```python
from build123d import *

# Parameters (mm, degrees)
SKETCH2_R      = 12.7
EXTRUDE1_DEPTH = 12.7


with BuildPart() as part:
    # Sketch2 → Extrude1 (new, symmetric)
    with BuildSketch(Plane.XY):
        Polygon((0, -28.575), (0, -66.675), (76.2, -85.725), (76.2, -123.825), (-114.3, -123.825), (-114.3, -85.725), (-38.1, 28.575), (28.575, 28.575), (28.575, -28.575), align=None)
        with Locations(Location((0, 0, 0), (0, 0, 180))):
            Circle(SKETCH2_R, mode=Mode.SUBTRACT)
    extrude(amount=EXTRUDE1_DEPTH, both=True)


solid = part.part
```
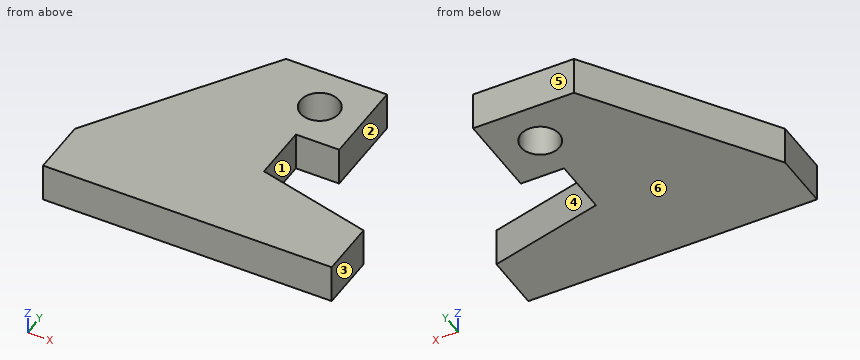
Design review of the part built by this model. Coordinates are the model's own, in mm. Face numbers are marked on the shaded views. A direction names the side the tool comes from. Give positions to 0.01 mm unless a question says otherwise; leave off trailing zeros. Order: outer loops, then holes, each group sorted by start corner. A loop starts at its lowest first (then second) coordinate and runs counter-clockwise, first axis right, second up. Notation, with made-up numbers: (-30, 63) -> (28, 63) arc R13 cw to (28, 67) -> close; hole circle Ø3 at (-36, 22). An arc over 180 degrees is marked (long way). Write item = value, one per line. Start each with the question number.
(1) We need section C-C on x = -4.5. Write out the cut boundary in (y, z) (3 decimals), plus the area to 3 significant figures.
(2) We need section D-D on y = -75. Write out the cut boundary in (x, z).
(3) To check wall thickness, follow line 1 along X through (y, z) = (2, 2.25) (3 decimals); line 2 along X through (y, z) = (7, -2.25) (3 decimals); line 3 along Y through (x, z) = (-94, 0) (3 decimals). State the ranges of each line that lie inside material, in increasing order.
(4) We need section A-A on z = 9.75. Write out the cut boundary in (x, y) (3 decimals).
(5) Mouldability with a two-part tool opening along Y and no side actions: class the marked faces 4, 5 and 6 as +Y half, -Y half, draft (parallel to the pull), parting line (faces both ways), or undercut.
(6) For the marked faces 1, 2 and 3, list the 3-axis set-ups (+Z, -Z, +X, -X, +Y, -Y) from which the entire face can be reached by the end or side of a thin tool; tool diameter is ignored.
(7) We need section B-B on y = 0. Write out the cut boundary in (x, z) (3 decimals), plus the area to 3 significant figures.
(8) For pin 1 (12 mm diameter, centred on x = -75.5, z = -3, fed in from +Y) (3 decimals); pin 2 (2 mm diameter, centred on y = -55, z = 3, fed in from -X); pin 3 (1.5 mm diameter, centred on x = -54, z = 10, fed in from +Y), all flat-tipped, find the tip position at first contact; note any pin that passes through.
Numbers:
q1.outline = (-123.825, -12.7) -> (-11.876, -12.7) -> (-11.876, 12.7) -> (-123.825, 12.7) -> close; (11.876, -12.7) -> (28.575, -12.7) -> (28.575, 12.7) -> (11.876, 12.7) -> close
q1.area = 3,270 mm^2
q2.outline = (-107.15, -12.7) -> (33.3, -12.7) -> (33.3, 12.7) -> (-107.15, 12.7) -> close
q3.line_1 = -55.817 to -12.542, 12.542 to 28.575
q3.line_2 = -52.483 to -10.597, 10.597 to 28.575
q3.line_3 = -123.825 to -55.275
q4.outline = (-114.3, -123.825) -> (76.2, -123.825) -> (76.2, -85.725) -> (0, -66.675) -> (0, -28.575) -> (28.575, -28.575) -> (28.575, 28.575) -> (-38.1, 28.575) -> (-114.3, -85.725) -> close; hole circle Ø25.4 at (0, 0)
q5.face_4 = undercut
q5.face_5 = +Y half
q5.face_6 = draft
q6.face_1 = +Z, -Z, +X
q6.face_2 = +Z, -Z, +X, +Y
q6.face_3 = +Z, -Z, +X, +Y, -Y
q7.outline = (-57.15, -12.7) -> (-12.7, -12.7) -> (-12.7, 12.7) -> (-57.15, 12.7) -> close; (12.7, -12.7) -> (28.575, -12.7) -> (28.575, 12.7) -> (12.7, 12.7) -> close
q7.area = 1,530 mm^2
q8.pin_1 = -18.525
q8.pin_2 = -94.48
q8.pin_3 = 5.85
